```python
from build123d import *

# Parameters (mm, degrees)
BOSS_EXTRUDE1_DEPTH = 12


with BuildPart() as part:
    # Sketch2 → Revolve1 (revolve)
    with BuildSketch(Plane.XY.offset(-57), mode=Mode.PRIVATE) as revolve1_sk:
        with BuildLine():
            Line((-12, 115), (12, 115))
            Line((12, 115), (12, 124))
            ThreePointArc((12, 124), (9.421572875, 125.275126266), (8.5, 128))
            Line((8.5, 128), (-8.5, 128))
            ThreePointArc((-8.5, 128), (-9.421572875, 125.275126266), (-12, 124))
            Line((-12, 124), (-12, 115))
        make_face()
    revolve(revolve1_sk.sketch.rotate(Axis((-36.047482345, 104, -57), (1, 0, 0)), 90), axis=Axis((-36.047482345, 104, -57), (1, 0, 0)))

    # Sketch3 → Boss-Extrude1 (add, symmetric)
    with BuildSketch(Plane(origin=(0, 0, 0), x_dir=(0, 0, -1), z_dir=(1, 0, 0))):
        with BuildLine():
            Line((0, 0), (0, 87))
            Line((0, 87), (41.444008538, 122.275971373))
            ThreePointArc((41.444008538, 122.275971373), (40.02971958, 87.029154927), (75.276488949, 88.444616633))
            Line((75.276488949, 88.444616633), (0, 0))
        make_face()
    extrude(amount=BOSS_EXTRUDE1_DEPTH, both=True)


solid = part.part
```
Input: part model. Units: mm. Frame: model coordinates. A direction names the side the tool comes from. Give positions to 0.01 mm unless a question says otherwise; leave off trailing zeros. Loops run counter-clockwise (first coordinate to the right, second up) from the corner with the lowest first, then second, coordinate; pieces in that order, holes last. Notation, with made-up numbers: M 34,-6.75 L 38,-6.75 A29 ccw 38,17.25 Z; hole C 3,-20 d2. An arc over 180 degrees is marked long. Answer as CSV lines item,"result". Start each with the question number.
1. Section B-B on y = 104. Return loops of the section in (x, z).
2. Section D-D on y = 64. Return loops of the section in (x, z).
3. Pin query (flat end, axial travel): P1, Ø6, axis at y = 76, z = -65, coming from the +X side; P2, Ø8, axis at x = 8.5, y = 96, coming from the +Z side; P3, Ø6, axis at x = -9.5, z = -40, coming from the -Y side; P4, Ø4, axis at x = 9.5, y = 25, coming from the -Z side. Return the tip coordinate at first contact, or that it passes through.
4. Line query: L1, parallel to Z at x = 9.25, y = 104; L2, parallel to Z at x = -9.35, y = 104; L3, parallel to Y at x = 11.25, z = -52. Output: solid intervals per line, ascending.
5. Reachability of faces 1 (the face through (-12, 113, -48)), 2 (the face through (-10.23, 87.43, -39.64)) from +Z, -Z, +X, -X, +Y, -Y: full face, straight path, thin tool, end or side. Return the list, or none.
6. Pull-direction query (Y, two-part tool) for faces 3 (the face through (-12, 62, -21)), 4 (the face through (10.27, 87.43, -39.64)), 5 (the face through (0.168, 44.841, -38.165)); classes: released by +Y, released by -Y, zero draft, split by the parting line, or undercut.
7. Section A-A on z = -57. Return loops of the section in (x, y).
8. Section C-C on x = 1.5. Return loops of the section in (y, z), plus the area to 3 significant figures.
Computed values:
1,outline,"M -12,-77 A3.76 cw -8.5,-81 L 8.5,-81 A3.76 cw 12,-77 L 12,-68 L -12,-68 Z; M -12,-46 L 12,-46 L 12,-37 A3.76 cw 8.5,-33 L 12,-33 L 12,-19.97 L -12,-19.97 L -12,-33 L -8.5,-33 A3.76 cw -12,-37 Z"
2,outline,"M -12,-54.47 L 12,-54.47 L 12,0 L -12,0 Z"
3,P1,"stops at x = 12"
3,P2,"stops at z = -5.87"
3,P3,"stops at y = 43.47"
3,P4,"stops at z = -22.98"
4,L1,"z = -78.49 to -68, -46 to -35.51, -33 to -19.97"
4,L2,"z = -78.36 to -68, -46 to -35.64, -33 to -19.97"
4,L3,"y = 61.1 to 80.53, 84.5 to 94.2, 113.8 to 123.5"
5,face 1,"+Z, -Z, -X, +Y, -Y"
5,face 2,"-X"
6,face 3,"zero draft"
6,face 4,"undercut"
6,face 5,"released by -Y"
7,outline,"M -12,66.97 L 12,66.97 L 12,80 L 8.5,80 A3.76 cw 12,84 L 12,93 L -12,93 L -12,84 A3.76 cw -8.5,80 L -12,80 Z; M -12,115 L 12,115 L 12,124 A3.76 cw 8.5,128 L -8.5,128 A3.76 cw -12,124 Z"
8,outline,"M 0,0 L 88.44,-75.28 A24 ccw 122.28,-41.44 L 87,0 Z; hole C 104,-57 d22"
8,area,"5,000 mm²"
